Verification items for this drawing (mm, ordinates from the low corner). A direction names the side the tool comes from. Round coordinates to 2 decimals unless told otherwise and drop trailing zeros. Order: outer loops, then holes, each group sorted by start corner. A loop starts at its lowest first (then second) coordinate and runs counter-clockwise, first axis right, second up. Notation, with made-up numbers: (-20.5, -1) -> (-4.5, -1) arc R15 ccw to (-4.5, 13) -> close; hole circle Ø4 at (42, -29). An arc over 180 degrees is marked (long way). Use a Markdown table: item, result. Add a question column.
Item 1: Sectioned sample at A-A, the plane y = 2.05. Record the cut outline in (x, z).
Item 2: Sectioned sample at D-D, the plane y = 4.1. Record the cut outline in (x, z), and give its area (3 significant figures).
Item 3: Sectioned sample at B-B, the plane z = 12.5. Record the cut outline in (x, y).
Item 4: Gauge pin test, flat ends, axial feed: pin 1 Ø1.6 at (y, z) = (2.5, 7.5) entering from -X; pin 2 Ø1.6 at (y, z) = (2.5, 8) entering from +X. Record the tip position at first contact, or that the pin passes through.
Item 5: Material ranges on probe 1 along Z at (x, y) = (6.25, 2.15); probe 2 along Z at (x, y) = (8.75, 2.1); probe 3 along X at (y, z) = (2.6, 10.75), recorded low to high. Write a range as [from, to].
Item 6: Sectioned sample at C-C, the plane x = 1.75. Record the cut outline in (y, z).
Item 7: Mould release check, pull along X, two halves, no side actions. Record for the marked faces 4, 5 and 6: pulls with the +X half, pulls with the -X half, needs draft (parallel to the pull), parting line crosses it, or undercut.
Item 8: Set-up check for the marked faces 1, 2 and 3: record each of +Z, -Z, +X, -X, +Y, -Y from which the full face is reachable in a straight line by a thin tool's end or side.
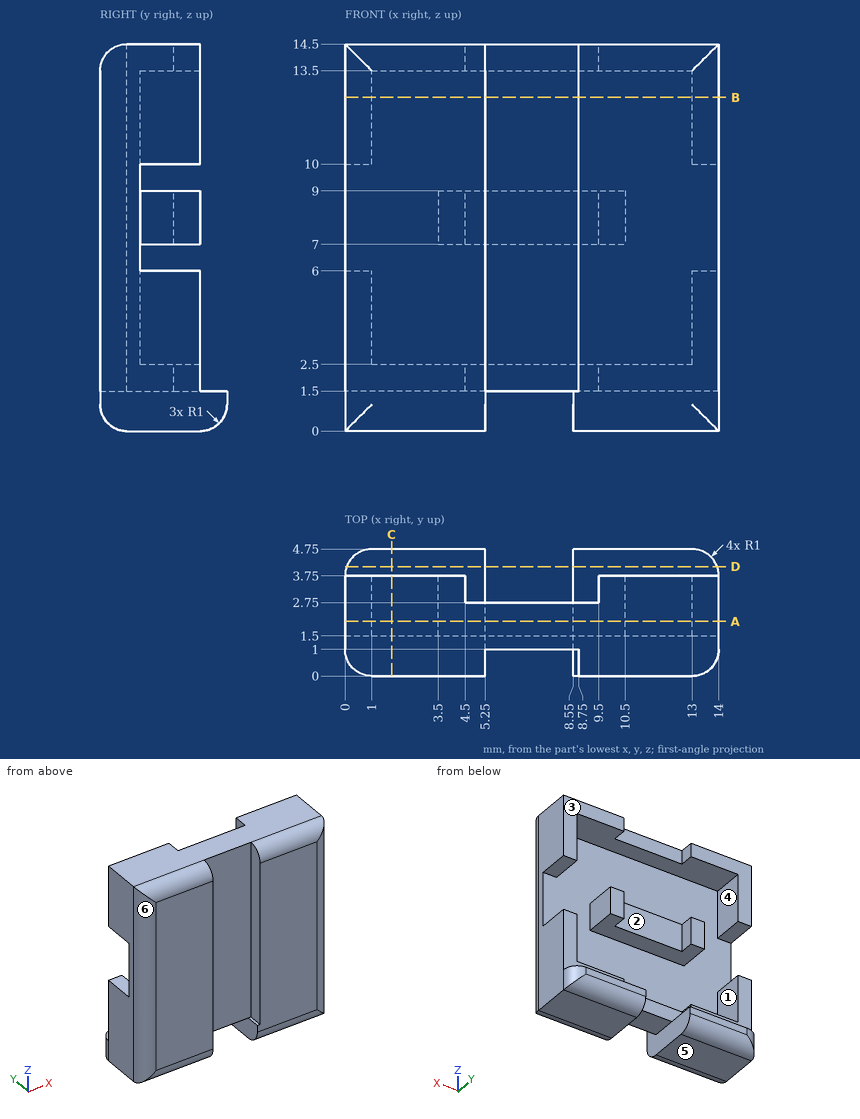
Found:
| question | item | result |
|---|---|---|
| 1 | outline | (0, 0) -> (5.25, 0) -> (5.25, 1.5) -> (8.55, 1.5) -> (8.55, 0) -> (14, 0) -> (14, 6) -> (13, 6) -> (13, 2.5) -> (1, 2.5) -> (1, 6) -> (0, 6) -> close; (0, 10) -> (1, 10) -> (1, 13.5) -> (13, 13.5) -> (13, 10) -> (14, 10) -> (14, 14.5) -> (0, 14.5) -> close; (3.5, 7) -> (10.5, 7) -> (10.5, 9) -> (3.5, 9) -> close |
| 2 | outline | (0.06, 0.06) -> (5.25, 0.06) -> (5.25, 1.5) -> (0.06, 1.5) -> close; (8.55, 0.06) -> (13.94, 0.06) -> (13.94, 1.5) -> (8.55, 1.5) -> close |
| 2 | area | 15.2 mm2 |
| 3 | outline | (0, 1) arc R1 ccw to (1, 0) -> (5.25, 0) -> (5.25, 1) -> (8.75, 1) -> (8.75, 0) -> (13, 0) arc R1 ccw to (14, 1) -> (14, 3.75) -> (13, 3.75) -> (13, 1.5) -> (1, 1.5) -> (1, 3.75) -> (0, 3.75) -> close |
| 4 | pin 1 | stops at x = 3.5 |
| 4 | pin 2 | stops at x = 10.5 |
| 5 | probe 1 | z = [1.5, 2.5], [7, 9], [13.5, 14.5] |
| 5 | probe 2 | z = [0, 2.5], [7, 9], [13.5, 14.5] |
| 5 | probe 3 | x = [0, 1], [13, 14] |
| 6 | outline | (0, 1) arc R1 ccw to (1, 0) -> (3.75, 0) arc R1 ccw to (4.75, 1) -> (4.75, 1.5) -> (3.75, 1.5) -> (3.75, 2.5) -> (1.5, 2.5) -> (1.5, 13.5) -> (3.75, 13.5) -> (3.75, 14.5) -> (1, 14.5) arc R1 ccw to (0, 13.5) -> close |
| 7 | face 4 | undercut |
| 7 | face 5 | needs draft |
| 7 | face 6 | pulls with the -X half |
| 8 | face 1 | +Y |
| 8 | face 2 | +Z, +Y |
| 8 | face 3 | +Z, +X, -X, +Y |
